Can you work these out from the model? Positions are in its coordinate system, mm. A direction names the side the tool comes from. Give positions to 0.01 mm unless a question says otherwise; leave off trailing zeros. Loops run counter-clockwise (first coordinate to the right, second up) from the corner with the lowest first, then second, coordinate; pieces in that order, holes last. Notation, with made-up numbers: (-24, -1) - (11, -1) arc R7 ccw to (11, 8) - close; hole circle Ø7 at (6.25, 23). An arc over 180 degrees is marked (long way). Answer in a Markdown table with one row per item.
from build123d import *

# Parameters (mm, degrees)
CUT_EXTRUDE1_START = -1.25
CUT_EXTRUDE1_DEPTH = 1.25
CHAMFER1_SIZE      = 0.25


with BuildPart() as part:
    # Sketch1 → Revolve1 (revolve)
    with BuildSketch(Plane.XY):
        Polygon((0, 0), (0, 2.719337567), (0.6, 2.719337567), (0.6, 0.219337567), (0.85, 0.075), (0.85, -0.075), (0.6, -0.219337567), (0.6, -10.069337567), (0, -10.069337567), align=None)
    revolve(axis=Axis((0, 0, 0), (0, 1, 0)))

    # Sketch2 → Cut-Extrude1 (cut)
    with BuildSketch(Plane(origin=(0, 2.719337567, 0), x_dir=(1, 0, 0), z_dir=(0, 1, 0)).offset(CUT_EXTRUDE1_START)):
        with BuildLine():
            Line((0, 0.6), (0, -0.6))
            ThreePointArc((0, -0.6), (0.6, 0), (0, 0.6))
        make_face()
    extrude(amount=CUT_EXTRUDE1_DEPTH, mode=Mode.SUBTRACT)

    # Chamfer1
    chamfer1_edges = [part.edges().sort_by_distance(p)[0] for p in [
        (-0.6, -10.069337567, 0),
    ]]
    chamfer(chamfer1_edges, length=CHAMFER1_SIZE)


solid = part.part
Q1. On a 3-axis mill with a long thin cutter (end or side, diameter ignored), from which of +Z, -Z, +X, -X, +Y, -Y can I reach the whole of each face in a straight line? I mean faces 1 (the face through (-0.6, 1.2, 0)), 2 (the face through (0, 2, 0)), 3 (the face through (0.323, -5.087, -0.506)). Say none if no direction works.
Checked values:
| item | result |
|---|---|
| face 1 | +Y |
| face 2 | +Z, -Z, +X, +Y |
| face 3 | -Y |
Q2. Imagine slicing it at B-B, the plane y = 1.25. Write out the boundary of the cut face in (x, z), and give its area (3 significant figures).
Checked values:
| item | result |
|---|---|
| outline | circle Ø1.2 at (0, 0) |
| area | 1.13 mm² |
Q3. If I drill on line 1 (X direction, y = -6.75, z = 0); line 2 (Y direction, x = 0.1, z = -0.1), over which ranges is the centre line in solid material (lowest first)? Write a range as [from, to].
Checked values:
| item | result |
|---|---|
| line 1 | x = [-0.6, 0.6] |
| line 2 | y = [-10.07, 1.47] |
Q4. Imagine slicing it at A-A, the plane z = 0. Write out the boundary of the cut face in (x, y) (3 decimals).
Checked values:
| item | result |
|---|---|
| outline | (-0.85, -0.075) - (-0.6, -0.219) - (-0.6, -9.819) - (-0.35, -10.069) - (0.35, -10.069) - (0.6, -9.819) - (0.6, -0.219) - (0.85, -0.075) - (0.85, 0.075) - (0.6, 0.219) - (0.6, 1.469) - (0, 1.469) - (0, 2.719) - (-0.6, 2.719) - (-0.6, 0.219) - (-0.85, 0.075) - close |
